The listing builds one solid part. Answer for the finished solid, in the listing's coordinates (mm). A direction names the side the tool comes from. Round coordinates to 2 decimals unless told otherwise and drop trailing zeros. Loops run counter-clockwise (first coordinate to the right, second up) from the corner with the lowest first, then second, coordinate; pieces in that order, holes last. Notation, with made-up numbers: (1, 70) -> (12, 70) arc R27 ccw to (12, 106) -> close; hole circle Ø2 at (26.25, -26). An arc over 180 degrees is marked (long way). Use a Markdown table: item, result. Add a question column.
Q1. Section C-C on z = 0 is taken. Give the vertices of the cut face in (x, y), then the cut area to 3 significant figures.
Q2. Which of the six approach directions +Z, -Z, +X, -X, +Y, -Y give full straight-line access (tool end or side, diameter ignored) to faces 5 (the flat face through (-1, 8, 5)), 6 (the flat face through (17, 20, 2)), 7 (the cylindrical face through (0.9, 2.96, -2.86))?
Q3. Section B-B on x = 30 is taken. Give the vertices of the cut face in (y, z).
Q4. Section A-A on y = 4 is taken. Give the vertices of the cut face in (x, z), then the cut area to 3 significant figures.
Q5. Section D-D on x = -1 is taken. Give the vertices of the cut face in (y, z), then the cut area to 3 significant figures.
Q6. For a pull along X with two mould halves and no side action, classify faces 1 (the flat face through (37.5, 11, 0)), 2 (the flat face through (-37.5, 11, 0)), 3 (the cylindrical face through (-27.106, 23.486, 1.135)), 4 (the flat face through (-25, 6, 0)) as released by +X, released by -X, zero draft, split by the parting line, or undercut.
Q7. Consider line 1 (X direction, y = 4.5, z = 0); line 2 (X direction, y = 18, z = -3); line 3 (Y direction, x = 3, z = 4.5). Determine where each line is inside the solid, lowest interval first.
Q8. Given pin 1 Ø1.5 at (x, y) = (-2.5, 15) entering from +Z; pin 2 Ø6 at (x, z) = (-11.5, -1.5) entering from +Y; pin 3 Ø3 at (x, z) = (-0.5, 0) entering from -Y, each flat-ended and moving along its own axis, determine where each tip first touches the part or whether it passes through.
from build123d import *

# Parameters (mm, degrees)
CROQUIS1_W              = 75
CROQUIS1_H              = 10
SALIENTE_EXTRUIR1_DEPTH = 15
SALIENTE_EXTRUIR2_DEPTH = 75
CROQUIS3_W              = 34
CROQUIS3_H              = 20.463300895
CORTAR_EXTRUIR1_DEPTH   = 53
CROQUIS4_R              = 3
CORTAR_EXTRUIR2_DEPTH   = 82
CROQUIS5_R              = 3
CORTAR_EXTRUIR3_DEPTH   = 6


with BuildPart() as part:
    # Croquis1 → Saliente-Extruir1 (new body)
    with BuildSketch(Plane(origin=(0, 0, 0), x_dir=(1, 0, 0), z_dir=(0, 1, 0))):
        Rectangle(CROQUIS1_W, CROQUIS1_H)
    extrude(amount=SALIENTE_EXTRUIR1_DEPTH)

    # Croquis2 → Saliente-Extruir2 (add)
    with BuildSketch(Plane.ZY.offset(37.5)):
        with BuildLine():
            Line((-5, 15), (5, 15))
            Line((5, 15), (5, 16.974190569))
            ThreePointArc((5, 16.974190569), (5.365546157, 18.409339673), (6.373101968, 19.494746617))
            Line((6.373101968, 19.494746617), (7.318770394, 20.105130227))
            ThreePointArc((7.318770394, 20.105130227), (8.653897933, 22.149866442), (8.026350555, 24.509886785))
            Line((8.026350555, 24.509886785), (6.189450494, 26.785760885))
            ThreePointArc((6.189450494, 26.785760885), (3.846087211, 27.901547218), (1.509374249, 26.77189986))
            Line((1.509374249, 26.77189986), (-4.34559805, 19.429162497))
            ThreePointArc((-4.34559805, 19.429162497), (-4.831677431, 18.549581775), (-5, 17.558823013))
            Line((-5, 17.558823013), (-5, 15))
        make_face()
    extrude(amount=-SALIENTE_EXTRUIR2_DEPTH)

    # Croquis3 → Cortar-Extruir1 (cut)
    with BuildSketch(Plane(origin=(0, 0, -5), x_dir=(-1, 0, 0), z_dir=(0, 0, -1))):
        with Locations((0, 27.901560376)):
            Rectangle(CROQUIS3_W, CROQUIS3_H)
    extrude(amount=-CORTAR_EXTRUIR1_DEPTH, mode=Mode.SUBTRACT)

    # Croquis4 → Cortar-Extruir2 (cut)
    with BuildSketch(Plane(origin=(37.5, 0, 0), x_dir=(0, 0, -1), z_dir=(1, 0, 0))):
        with Locations((-3.996707054, 22.584588981)):
            Circle(CROQUIS4_R)
    extrude(amount=-CORTAR_EXTRUIR2_DEPTH, mode=Mode.SUBTRACT)

    # Croquis5 → Cortar-Extruir3 (cut)
    with BuildSketch(Plane.XZ):
        with Locations(Location((0, 0, 0), (0, 0, 270))):
            Circle(CROQUIS5_R)
        with Locations(Location((25, 0, 0), (0, 0, 270))):
            Circle(CROQUIS5_R)
        with Locations(Location((-25, 0, 0), (0, 0, 270))):
            Circle(CROQUIS5_R)
    extrude(amount=-CORTAR_EXTRUIR3_DEPTH, mode=Mode.SUBTRACT)


solid = part.part
Checked values:
| question | item | result |
|---|---|---|
| 1 | outline | (-37.5, 0) -> (-28, 0) -> (-28, 6) -> (-22, 6) -> (-22, 0) -> (-3, 0) -> (-3, 6) -> (3, 6) -> (3, 0) -> (22, 0) -> (22, 6) -> (28, 6) -> (28, 0) -> (37.5, 0) -> (37.5, 24.88) -> (17, 24.88) -> (17, 17.67) -> (-17, 17.67) -> (-17, 24.88) -> (-37.5, 24.88) -> close |
| 1 | area | 1,510 mm2 |
| 2 | face 5 | +Z, +X, -X, -Y |
| 2 | face 6 | +Z, -Z, +Y |
| 2 | face 7 | -Y |
| 3 | outline | (0, -5) -> (17.56, -5) arc R3 ccw to (19.43, -4.35) -> (26.77, 1.51) arc R3 ccw to (26.79, 6.19) -> (24.51, 8.03) arc R3 ccw to (20.11, 7.32) -> (19.49, 6.37) arc R3 cw to (16.97, 5) -> (0, 5) -> close; hole circle Ø6 at (22.58, 4) |
| 4 | outline | (-37.5, -5) -> (37.5, -5) -> (37.5, 5) -> (-37.5, 5) -> close; hole circle Ø6 at (-25, 0); hole circle Ø6 at (0, 0); hole circle Ø6 at (25, 0) |
| 4 | area | 665 mm2 |
| 5 | outline | (0, -5) -> (17.56, -5) arc R3 ccw to (17.67, -5) -> (17.67, 5.08) arc R3 cw to (16.97, 5) -> (0, 5) -> (0, 2.83) -> (6, 2.83) -> (6, -2.83) -> (0, -2.83) -> close |
| 5 | area | 143 mm2 |
| 6 | face 1 | released by +X |
| 6 | face 2 | released by -X |
| 6 | face 3 | zero draft |
| 6 | face 4 | undercut |
| 7 | line 1 | x = -37.5 to -28, -22 to -3, 3 to 22, 28 to 37.5 |
| 7 | line 2 | x = -37.5 to -17, 17 to 37.5 |
| 7 | line 3 | y = 0 to 17.67 |
| 8 | pin 1 | stops at z = 5 |
| 8 | pin 2 | stops at y = 17.67 |
| 8 | pin 3 | stops at y = 6 |
